from build123d import *

# Parameters (mm, degrees)
SKETCH1_R             = 11
SKETCH1_R_2           = 5
BOSS_EXTRUDE1_DEPTH   = 4
SKETCH2_R             = 9.5
SKETCH2_R_2           = 6.75
CUT_EXTRUDE1_DEPTH    = 0.1
MIRROR1_START         = -4
MIRROR1_OUTLINE_R     = 9.5
MIRROR1_OUTLINE_R_2   = 6.75
MIRROR1_DEPTH         = 0.1
MIRROR1_START_2       = 3.8
MIRROR1_2_OUTLINE_R   = 9.5
MIRROR1_2_OUTLINE_R_2 = 6.75
MIRROR1_2_DEPTH       = 0.1
FILLET1_R             = 0.3


# Read off the part's stored shape, not the designer's step: Mirror1
with BuildPart() as part:
    # Sketch1 → Boss-Extrude1 (new, symmetric)
    with BuildSketch(Plane.XY):
        Circle(SKETCH1_R)
        Circle(SKETCH1_R_2, mode=Mode.SUBTRACT)
    extrude(amount=BOSS_EXTRUDE1_DEPTH, both=True)

    # Sketch2 → Cut-Extrude1 (cut)
    with BuildSketch(Plane.XY.offset(4)):
        Circle(SKETCH2_R)
        Circle(SKETCH2_R_2, mode=Mode.SUBTRACT)
    extrude(amount=-CUT_EXTRUDE1_DEPTH, mode=Mode.SUBTRACT)

    # Mirror1 outline → Mirror1 (cut)
    with BuildSketch(Plane.XY.offset(MIRROR1_START)):
        Circle(MIRROR1_OUTLINE_R)
        Circle(MIRROR1_OUTLINE_R_2, mode=Mode.SUBTRACT)
    extrude(amount=MIRROR1_DEPTH, mode=Mode.SUBTRACT)

    # Mirror1 2 outline → Mirror1 2 (cut)
    with BuildSketch(Plane.XY.offset(MIRROR1_START_2)):
        Circle(MIRROR1_2_OUTLINE_R)
        Circle(MIRROR1_2_OUTLINE_R_2, mode=Mode.SUBTRACT)
    extrude(amount=MIRROR1_2_DEPTH, mode=Mode.SUBTRACT)

    # Fillet1
    fillet1_edges = [part.edges().sort_by_distance(p)[0] for p in [
        (-11, 0, -4),
        (-11, 0, 4),
        (-5, 0, -4),
        (-5, 0, 4),
    ]]
    fillet(fillet1_edges, radius=FILLET1_R)


solid = part.part
Input: part model. Units: mm. Frame: model coordinates. A direction names the side the tool comes from. Coordinates: 2 decimals unless noted, no trailing zeros. Order: outer loops, then holes, each group sorted by start corner. A loop starts at its lowest first (then second) coordinate and runs counter-clockwise, first axis right, second up. Notation, with made-up numbers: M -10,38 L -5,38 A12 ccw -5,52 Z; hole C 17,14.5 d5. An arc over 180 degrees is marked long. Write item = value, one per line. Start each with the question number.
(1) Line query: line 1 along Y through (x, z) = (-4.25, -2.75); line 2 along Y through (x, z) = (0, 3.95); line 3 along Y through (x, z) = (0, -3.85). Output: solid intervals per line, ascending. Write a range as [from, to].
(2) Reachability of faces 5 (the flat face through (4, -6, -3.9)), 6 (the flat face through (0, 10, -4)) from +Z, -Z, +X, -X, +Y, -Y: full face, straight path, thin tool, end or side. Return the list, or none.
(3) Section C-C on z = 2. Output: boundary loops of the cut face in (x, y), and give its area (3 significant figures).
(4) Pull-direction query (Y, two-part tool) for faces 1 (the cylindrical face through (-2.38, -10.74, 0.05)), 2 (the flat face through (4, -6, 3.8)), 3 (the flat face through (-5, -3, -4)), 4 (the cylindrical face through (-1.08, -4.88, -0.05)); classes: released by +Y, released by -Y, zero draft, split by the parting line, or undercut.
(5) First-contact query: P1, Ø1, axis at x = -6.5, z = -2.5, coming from the +Y side; P2, Ø3, axis at x = -6, z = -1, coming from the -Y side; P3, Ø1, axis at x = 3, z = -3, coming from the -Y side. Flat tips, straight axial feed; report the tip coordinate or a pass-through.
Result set:
q1.line_1 = [-10.15, -2.63], [2.63, 10.15]
q1.line_2 = [-10.87, -9.5], [-6.75, -5.13], [5.13, 6.75], [9.5, 10.87]
q1.line_3 = [-10.96, -5.04], [5.04, 10.96]
q2.face_5 = -Z
q2.face_6 = -Z, +X, -X, +Y, -Y
q3.outline = C 0,0 d22; hole C 0,0 d10
q3.area = 302 mm²
q4.face_1 = split by the parting line
q4.face_2 = undercut
q4.face_3 = zero draft
q4.face_4 = undercut
q5.P1 = 9.22
q5.P2 = -10.04
q5.P3 = -10.71
